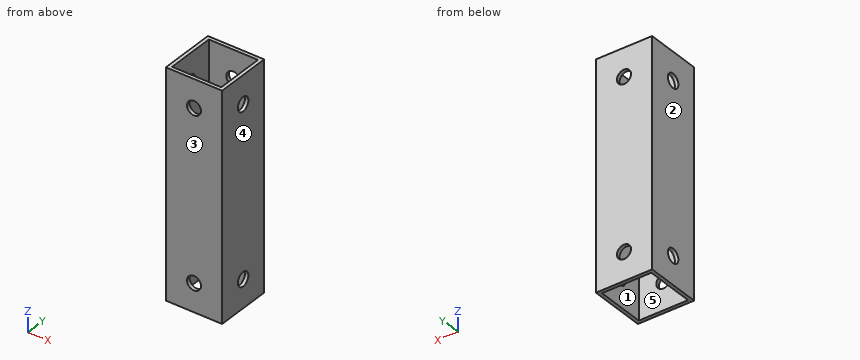
Autodesk Inventor part; units mm, degrees
ref_plane "YZ Plane" through (0, 0, 0) normal (1, 0, 0) x (0, 1, 0)
ref_plane "XZ Plane" through (0, 0, 0) normal (0, 1, 0) x (-1, 0, 0)
ref_plane "XY Plane" through (0, 0, 0) normal (0, 0, 1) x (1, 0, 0)
sketch "Sketch1" plane through (0, 0, 0) normal (0, 0, 1) x (1, 0, 0)
  line L0 (0, 0) -> (25.4, 0)
  line L1 (25.4, 0) -> (25.4, 25.4)
  line L2 (25.4, 25.4) -> (0, 25.4)
  line L3 (0, 25.4) -> (0, 0)
  line L4 (1.5875, 23.8125) -> (23.8125, 23.8125)
  line L5 (23.8125, 23.8125) -> (23.8125, 1.5875)
  line L6 (23.8125, 1.5875) -> (1.5875, 1.5875)
  line L7 (1.5875, 1.5875) -> (1.5875, 23.8125)
  dimension "d0" = 25.4
  dimension "d1" = 25.4
  dimension "d2" = 1.5875
extrude "Extrusion1" add sketch "Sketch1" against normal blind 101.6
sketch "Sketch2" plane through (25.4, 0, 0) normal (1, 0, 0) x (0, 0, -1)
  line L0 (101.6, 0) -> (101.6, 25.4)
  line L1 (0, 0) -> (0, 25.4)
  point P0 (12.7, 12.7)
  point P1 (88.9, 12.7)
  dimension "d5" = 12.7
  dimension "d6" = 12.7
sketch "Sketch3" plane through (0, 0, 0) normal (0, -1, 0) x (1, 0, 0)
  line L0 (0, -101.6) -> (25.4, -101.6)
  line L1 (0, 0) -> (25.4, 0)
  point P0 (12.7, -12.7)
  point P1 (12.7, -88.9)
  dimension "d7" = 12.7
  dimension "d8" = 12.7
hole "Hole1" at (25.4, 12.7, -12.7) at (25.4, 12.7, -88.9) direction (-1, 0, 0) diameter 6.35 depth 25.4 tip angle 118
hole "Hole2" at (12.7, 0, -12.7) at (12.7, 0, -88.9) direction (0, 1, 0) diameter 6.35 depth 25.4 tip angle 118
properties part number "1tube_4_layer1_outside"
For this review, take the finished solid that the model builds, in its own axes (mm). Face numbers are marked on the shaded views. A direction names the side the tool comes from. Give positions to 0.01 mm unless a question says otherwise; leave off trailing zeros. Write each loop counter-clockwise with the first axis right and the second up, starting at its lowest first coordinate (ties: lowest second). Pieces come first, ordered by that corner, then holes.
Item 1: The part is to be moulded in two halves that separate along X. For the marked faces 1, 2 and 3, say which applies: +X half, -X half, draft (parallel to the pull), parting line (faces both ways), or undercut.
Item 2: Take a section at B-B (z = -83.5). Give the boundary of the cut face in (x, y).
Item 3: Machinability: for the marked faces 4 and 5, which of the approach directions +Z, -Z, +X, -X, +Y, -Y give a long, thin tool a straight path to every point of the face, cutting with its end or side? Answer none if there is none.
Item 4: Take a section at A-A (x = 12.7). Give the boundary of the cut face in (y, z) (1 decimal).
Item 5: Wall thickness on probe 1 along Z at (x, y) = (12.7, 24.55) (3 decimals); probe 2 along X at (y, z) = (24.2, -12.7) (3 decimals); probe 3 along X at (y, z) = (9, -16): over which ranges is each line inside the solid? List them lowest first.
Item 6: Insertion check: P1, Ø4, axis at x = 12.7, z = -88.9, coming from the +Y side. The pin has a flat end and moves straight along its axis. Give the tip position at first contact, or say it passes through.
Item 7: Take a section at C-C (x = 7.75). Give the boundary of the cut face in (y, z).
Established:
1. face 1: undercut
1. face 2: -X half
1. face 3: draft
2. outline: (0, 0) - (25.4, 0) - (25.4, 25.4) - (0, 25.4) - close; hole (1.59, 1.59) - (23.81, 1.59) - (23.81, 23.81) - (1.59, 23.81) - close
3. face 4: +Z, -Z, +X, +Y, -Y
3. face 5: +Z, -Z
4. outline: (0, -101.6) - (1.6, -101.6) - (1.6, -92.1) - (0, -92.1) - close; (0, -85.7) - (1.6, -85.7) - (1.6, -15.9) - (0, -15.9) - close; (0, -9.5) - (1.6, -9.5) - (1.6, 0) - (0, 0) - close; (23.8, -101.6) - (25.4, -101.6) - (25.4, -92.1) - (23.8, -92.1) - close; (23.8, -85.7) - (25.4, -85.7) - (25.4, -15.9) - (23.8, -15.9) - close; (23.8, -9.5) - (25.4, -9.5) - (25.4, 0) - (23.8, 0) - close
5. probe 1: z = -101.6 to -92.075, -85.725 to -15.875, -9.525 to 0
5. probe 2: x = 0 to 9.525, 15.875 to 25.4
5. probe 3: x = 0 to 1.59, 23.81 to 25.4
6. P1: passes through
7. outline: (0, -101.6) - (1.59, -101.6) - (1.59, 0) - (0, 0) - close; (23.81, -101.6) - (25.4, -101.6) - (25.4, 0) - (23.81, 0) - close
